```python
from build123d import *

# Parameters (mm, degrees)
SKETCH1_R           = 40
BOSS_EXTRUDE1_DEPTH = 1.2
CUT_EXTRUDE1_REACH  = 58.581
SKETCH2_R           = 7.75
CUT_EXTRUDE2_REACH  = 58.581
SKETCH4_R           = 38.3
BOSS_EXTRUDE2_DEPTH = 5
SKETCH5_R           = 36.85
CUT_EXTRUDE3_DEPTH  = 5


with BuildPart() as part:
    # Sketch1 → Boss-Extrude1 (new body)
    with BuildSketch(Plane.XY):
        Circle(SKETCH1_R)
    extrude(amount=BOSS_EXTRUDE1_DEPTH)

    # Sketch2 → Cut-Extrude1 (cut, up to next)
    with BuildSketch(Plane.XY.offset(1.2), mode=Mode.PRIVATE) as cut_extrude1_sk1:
        with Locations((25, 0)):
            Circle(SKETCH2_R)
    cut_extrude1_tool1 = extrude(cut_extrude1_sk1.sketch, amount=-CUT_EXTRUDE1_REACH, mode=Mode.PRIVATE) & part.part
    add(cut_extrude1_tool1.solids().sort_by_distance((25, 0, 1.2))[0], mode=Mode.SUBTRACT)

    # Sketch3 → Cut-Extrude2 (cut, up to next)
    with BuildSketch(Plane.XY.offset(1.2), mode=Mode.PRIVATE) as cut_extrude2_sk1:
        with BuildLine():
            Line((-27.5, 5), (-12.5, 5))
            ThreePointArc((-12.5, 5), (-7.5, 0), (-12.5, -5))
            Line((-12.5, -5), (-27.5, -5))
            ThreePointArc((-27.5, -5), (-32.5, 0), (-27.5, 5))
        make_face()
    cut_extrude2_tool1 = extrude(cut_extrude2_sk1.sketch, amount=-CUT_EXTRUDE2_REACH, mode=Mode.PRIVATE) & part.part
    add(cut_extrude2_tool1.solids().sort_by_distance((-20, 0, 1.2))[0], mode=Mode.SUBTRACT)

    # Sketch4 → Boss-Extrude2 (add)
    with BuildSketch(Plane.XY.offset(1.2)):
        Circle(SKETCH4_R)
    extrude(amount=BOSS_EXTRUDE2_DEPTH)

    # Sketch5 → Cut-Extrude3 (cut)
    with BuildSketch(Plane.XY.offset(6.2)):
        Circle(SKETCH5_R)
    extrude(amount=-CUT_EXTRUDE3_DEPTH, mode=Mode.SUBTRACT)


solid = part.part
```
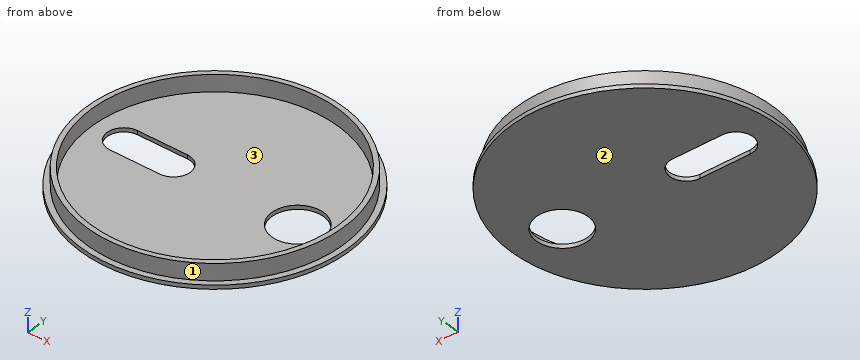
The model under review builds one solid part; all positions refer to its coordinate system, in mm. Face numbers are marked on the shaded views. Round coordinates to 2 decimals unless told otherwise and drop trailing zeros. Loops run counter-clockwise (first coordinate to the right, second up) from the corner with the lowest first, then second, coordinate; pieces in that order, holes last.
1) Consider section A-A on y = 0. State the section outline as (x, z) points.
Values follow:
outline: (-40, 0) - (-32.5, 0) - (-32.5, 1.2) - (-36.85, 1.2) - (-36.85, 6.2) - (-38.3, 6.2) - (-38.3, 1.2) - (-40, 1.2) - close; (-7.5, 0) - (17.25, 0) - (17.25, 1.2) - (-7.5, 1.2) - close; (32.75, 0) - (40, 0) - (40, 1.2) - (38.3, 1.2) - (38.3, 6.2) - (36.85, 6.2) - (36.85, 1.2) - (32.75, 1.2) - close
2) Consider section C-C on x = 23.5. State the section outline as (y, z) points, then the cut area to 3 significant figures.
Values follow:
outline: (-32.37, 0) - (-7.6, 0) - (-7.6, 1.2) - (-28.38, 1.2) - (-28.38, 6.2) - (-30.24, 6.2) - (-30.24, 1.2) - (-32.37, 1.2) - close; (7.6, 0) - (32.37, 0) - (32.37, 1.2) - (30.24, 1.2) - (30.24, 6.2) - (28.38, 6.2) - (28.38, 1.2) - (7.6, 1.2) - close
area: 78.0 mm2
3) Consider section D-D on z = 2.25. State the section outline as (x, y) points.
Values follow:
outline: circle Ø76.6 at (0, 0); hole circle Ø73.7 at (0, 0)
4) Consider section B-B on x = 0. State the section outline as (y, z) points.
Values follow:
outline: (-40, 0) - (40, 0) - (40, 1.2) - (38.3, 1.2) - (38.3, 6.2) - (36.85, 6.2) - (36.85, 1.2) - (-36.85, 1.2) - (-36.85, 6.2) - (-38.3, 6.2) - (-38.3, 1.2) - (-40, 1.2) - close
5) Clearance check with flat-ended pins moving along their axes: P1, Ø1.5, axis at x = -20, z = 1.5, coming from the -Y side; P2, Ø25, axis at x = 25, y = 0, coming from the +Z side; P3, Ø1.5, axis at y = -28, z = 2.5, coming from the -X side; P4, Ø1, axis at x = -22.5, z = 0.5, coming from the -Y side. State where each tip first meets the part, or that it passes through.
Values follow:
P1: stops at y = -35.03
P2: stops at z = 6.2
P3: stops at x = -26.91
P4: stops at y = -33.41
6) The part is to be moulded in two halves that separate along X. For the marked faces 1, 2 and 3, say which applies: pulls with the +X half, pulls with the -X half, needs draft (parallel to the pull), parting line crosses it, or undercut.
Values follow:
face 1: parting line crosses it
face 2: needs draft
face 3: undercut
7) Wall thickness on line 1 along Z through (x, y) = (2.5, -3); line 2 along Y through (x, z) = (-8.5, 5); line 3 along Y through (x, z) = (0, 3.9): over which ranges is each line inside the solid? List them lowest first.
Values follow:
line 1: z = 0 to 1.2
line 2: y = -37.34 to -35.86, 35.86 to 37.34
line 3: y = -38.3 to -36.85, 36.85 to 38.3
